from build123d import *

# Parameters (mm, degrees)
BOSS_EXTRUDE1_DEPTH      = 130.8
SKETCH5_R                = 10.65
CUT_EXTRUDE4_DEPTH       = 129.8
SKETCH6_R                = 10.65
CUT_EXTRUDE5_DEPTH       = 129.8
SKETCH57_R               = 10.7
CUT_EXTRUDE48_DEPTH      = 148.089829044
CUT_EXTRUDE51_DEPTH      = 132.35522197
CUT_EXTRUDE51_DEPTH_BACK = 132.35522197
SKETCH60_R               = 2
CUT_EXTRUDE52_DEPTH      = 132.574432074
CUT_EXTRUDE52_DEPTH_BACK = 132.574432074
SKETCH61_R               = 2.000000001
SKETCH63_R               = 1
CUT_EXTRUDE53_DEPTH      = 155.429604817
SKETCH64_R               = 1
CUT_EXTRUDE54_DEPTH      = 157.678735431
SKETCH65_R               = 1
CUT_EXTRUDE55_DEPTH      = 157.678735431
SKETCH66_R               = 1
CUT_EXTRUDE56_DEPTH      = 155.429604817


with BuildPart() as part:
    # Sketch1 → Boss-Extrude1 (new body)
    with BuildSketch(Plane(origin=(0, 0, 0), x_dir=(0.999872775920664, 0, 0.01595092388251422), z_dir=(0, 1, 0))):
        with BuildLine():
            Line((70.372282363, 4.818066557), (66.856282363, 4.818066557))
            ThreePointArc((66.856282363, 4.818066557), (4.002282363, -58.035933443), (-58.851717637, 4.818066557))
            Line((-58.851717637, 4.818066557), (-62.367717637, 4.818066557))
            ThreePointArc((-62.367717637, 4.818066557), (4.002282363, -61.551933443), (70.372282363, 4.818066557))
        make_face()
    extrude(amount=BOSS_EXTRUDE1_DEPTH)

    # Sketch5 → Cut-Extrude4 (cut)
    with BuildSketch(Plane(origin=(63.687908888, 47.899932993, -8.621348971), x_dir=(0.015950923882504298, 0, -0.9998727759206641), z_dir=(0.9998727759206643, 0, 0.015950923882504298))):
        with Locations((-4.818066557, 1.350067007)):
            Circle(SKETCH5_R)
    extrude(amount=CUT_EXTRUDE4_DEPTH, mode=Mode.SUBTRACT)

    # Sketch6 → Cut-Extrude5 (cut)
    with BuildSketch(Plane(origin=(-55.376952084, 47.899932993, -10.520785159), x_dir=(-0.01595092388248271, 0, 0.9998727759206645), z_dir=(-0.9998727759206645, 0, -0.01595092388248271))):
        with Locations((4.818066557, 49.750067007)):
            Circle(SKETCH6_R)
    extrude(amount=CUT_EXTRUDE5_DEPTH, mode=Mode.SUBTRACT)

    # Sketch57 → Cut-Extrude48 (cut, through all)
    with BuildSketch(Plane(origin=(-1.337515808, 38.899932993, 83.841265458), x_dir=(0.999872775920664, 0, 0.015950923882512152), z_dir=(-0.015950923882512152, 0, 0.999872775920664))):
        with Locations((4.002282363, 7.900067007)):
            Circle(SKETCH57_R)
    extrude(amount=-CUT_EXTRUDE48_DEPTH, mode=Mode.SUBTRACT)

    # Sketch60 → Cut-Extrude51 (cut, two sides: drawn at the far end of the back side and taken through both)
    with BuildSketch(Plane(origin=(4.479542792, 38.899932993, -4.33978545), x_dir=(0.6958141043149662, 0, 0.7182219240850013), z_dir=(-0.7182219240850013, 0, 0.6958141043149662)).offset(-CUT_EXTRUDE51_DEPTH_BACK)):
        with Locations(Location((-0.576184071, 87.550067007, 0), (0, 0, 180))):
            Circle(SKETCH60_R)
        with Locations(Location((-0.576184071, -34.599932993, 0), (0, 0, 180))):
            Circle(SKETCH60_R)
    extrude(amount=CUT_EXTRUDE51_DEPTH + CUT_EXTRUDE51_DEPTH_BACK, mode=Mode.SUBTRACT)

    # Sketch61 → Cut-Extrude52 (cut, two sides: drawn at the far end of the back side and taken through both)
    with BuildSketch(Plane(origin=(-0.400917003, 38.899932993, -0.413828032), x_dir=(0.7182219240850013, 0, -0.6958141043149662), z_dir=(0.6958141043149662, 0, 0.7182219240850013)).offset(-CUT_EXTRUDE52_DEPTH_BACK)):
        with Locations((6.236989769, 87.550067007)):
            Circle(SKETCH61_R)
        with Locations((6.236989769, -34.599932997)):
            Circle(SKETCH61_R)
    extrude(amount=CUT_EXTRUDE52_DEPTH + CUT_EXTRUDE52_DEPTH_BACK, mode=Mode.SUBTRACT)

    # Sketch63 → Cut-Extrude53 (cut, through all)
    with BuildSketch(Plane(origin=(48.51495843, 38.899932993, 50.087966302), x_dir=(0.718295826620825, 0, -0.6957378137338129), z_dir=(0.6957378137338129, 0, 0.718295826620825))):
        with Locations((-12.551102324, 15.400067007)):
            Circle(SKETCH63_R)
        with Locations((-12.551102324, 0.400067007)):
            Circle(SKETCH63_R)
    extrude(amount=-CUT_EXTRUDE53_DEPTH, mode=Mode.SUBTRACT)

    # Sketch64 → Cut-Extrude54 (cut, through all)
    with BuildSketch(Plane(origin=(-46.022353024, 38.899932993, 44.577025355), x_dir=(0.6957378137337953, 0, 0.7182958266208421), z_dir=(-0.7182958266208421, 0, 0.6957378137337953))):
        with Locations((18.069559284, 15.400067007)):
            Circle(SKETCH64_R)
        with Locations((18.069559284, 0.400067007)):
            Circle(SKETCH64_R)
    extrude(amount=-CUT_EXTRUDE54_DEPTH, mode=Mode.SUBTRACT)

    # Sketch65 → Cut-Extrude55 (cut, through all)
    with BuildSketch(Plane(origin=(-46.022353024, 38.899932993, 44.577025355), x_dir=(0.6957378137338341, 0, 0.7182958266208045), z_dir=(-0.7182958266208045, 0, 0.6957378137338341))):
        with Locations((-19.364877393, 66.250067007)):
            Circle(SKETCH65_R)
        with Locations((-19.364877393, 51.250067007)):
            Circle(SKETCH65_R)
    extrude(amount=-CUT_EXTRUDE55_DEPTH, mode=Mode.SUBTRACT)

    # Sketch66 → Cut-Extrude56 (cut, through all)
    with BuildSketch(Plane(origin=(48.51495843, 38.899932993, 50.087966302), x_dir=(0.7182958266208437, 0, -0.6957378137337936), z_dir=(0.6957378137337936, 0, 0.7182958266208437))):
        with Locations((24.883334353, 17.850067007)):
            Circle(SKETCH66_R)
        with Locations((24.883334353, 2.850067007)):
            Circle(SKETCH66_R)
    extrude(amount=-CUT_EXTRUDE56_DEPTH, mode=Mode.SUBTRACT)


solid = part.part
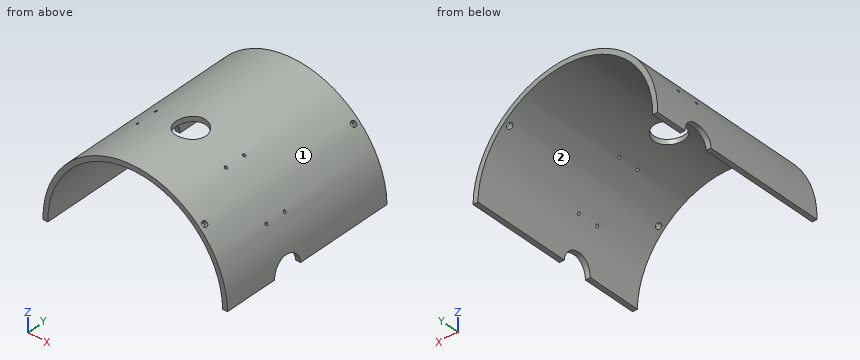
Verification items for the finished model (mm, model axes). Face numbers are marked on the shaded views. Coordinates: 2 decimals unless noted, no trailing zeros. Order: outer loops, then holes, each group sorted by start corner. A loop starts at its lowest first (then second) coordinate and runs counter-clockwise, first axis right, second up. Notation, with made-up numbers: M 25,-37 L 31,-37 A30 ccw 31,-15 Z; hole C 48,71.25 d3. An arc over 180 degrees is marked long. Return JSON: item names as keys, results as strings.
1) Cross-section at A-A, the plane z = 32. Record the boundary of the cut face in (x, y).
Answer list:
{"outline": "M -51.19,0 L -46.91,0 L -46.91,130.8 L -51.19,130.8 Z; M 55.07,0 L 59.34,0 L 59.34,130.8 L 55.07,130.8 Z"}
2) Thickness scan on L1, parallel to X at y = 23, z = 8; L2, parallel to X at y = 16.5, z = 46; L3, parallel to Z at x = 4, y = 66.5. Record the ranges inside material, lowest first. Write a range as [from, to].
Answer list:
{"L1": "[-61.05, -57.47], [65.63, 69.21]", "L2": "[-38.69, -33], [41.16, 46.85]", "L3": "[58.1, 61.62]"}
3) Cross-section at C-C, the plane z = 20. Record the boundary of the cut face in (x, y).
Answer list:
{"outline": "M -57.5,0 L -53.7,0 L -53.7,130.8 L -57.5,130.8 Z; M 61.85,0 L 65.66,0 L 65.66,130.8 L 61.85,130.8 Z"}
4) Cross-section at D-D, the plane x = -20.5. Record the boundary of the cut face in (y, z), and give its area (3 significant figures).
Answer list:
{"outline": "M 0,53.1 L 130.8,53.1 L 130.8,56.9 L 0,56.9 Z", "area": "497 mm2"}
5) Gauge pin test, flat ends, axial feed: pin 1 (1.5 mm diameter, centred on x = -36.5, z = 41, fed in from +Y); pin 2 (10 mm diameter, centred on x = 8.5, y = 53, fed in from -Z); pin 3 (10 mm diameter, centred on y = 99.5, z = 51.5, fed in from +X); pin 4 (10 mm diameter, centred on y = 109, z = 21, fed in from -X). Record the tip position at first contact, or that the pin passes through.
Answer list:
{"pin 1": "through", "pin 2": "z = 57.39", "pin 3": "x = 46.25", "pin 4": "x = -58.96"}
6) Release check for a two-part mould opening along X. For the marked faces 1 and 2 record: +X half, -X half, draft (parallel to the pull), parting line (faces both ways), or undercut.
Answer list:
{"face 1": "parting line", "face 2": "undercut"}
